from build123d import *

# Parameters (mm, degrees)
SCHIZZO4_R                   = 2.5
SCHIZZO4_R_2                 = 1.25
ESTRUSIONE_ESTRUSIONE3_DEPTH = 100
ESTRUSIONE_ESTRUSIONE4_DEPTH = 61.05
SCHIZZO6_W                   = 8.237008172
SCHIZZO6_H                   = 5.970383375
TAGLIO_ESTRUSIONE2_DEPTH     = 119.1
SCHIZZO7_W                   = 6.014694103
SCHIZZO7_H                   = 5.674261039
TAGLIO_ESTRUSIONE3_DEPTH     = 119.1
ESTRUSIONE_ESTRUSIONE5_REACH = 140.017
SCHIZZO8_W                   = 2.75
SCHIZZO8_H                   = 66.15
TAGLIO_ESTRUSIONE4_DEPTH     = 300
RACCORDO1_R                  = 2


with BuildPart() as part:
    # Schizzo4 → Estrusione-Estrusione3 (new body)
    with BuildSketch(Plane.XY):
        Circle(SCHIZZO4_R)
        Circle(SCHIZZO4_R_2, mode=Mode.SUBTRACT)
    extrude(amount=ESTRUSIONE_ESTRUSIONE3_DEPTH)

    # Schizzo5 → Estrusione-Estrusione4 (add, symmetric)
    with BuildSketch(Plane.XY.offset(50)):
        with BuildLine():
            Line((0, 2.5), (5, 2.5))
            Line((5, 2.5), (5, -64.15))
            Line((5, -64.15), (2.5, -64.15))
            Line((2.5, -64.15), (2.5, -2.5))
            Line((2.5, -2.5), (0, -2.5))
            ThreePointArc((0, -2.5), (2.5, 0), (0, 2.5))
        make_face()
    extrude(amount=ESTRUSIONE_ESTRUSIONE4_DEPTH, both=True)

    # Schizzo6 → Taglio-Estrusione2 (cut)
    with BuildSketch(Plane(origin=(0, 0, 0), x_dir=(-1, 0, 0), z_dir=(0, 0, -1))):
        with Locations((1.618504086, 0.485191688)):
            Rectangle(SCHIZZO6_W, SCHIZZO6_H)
    extrude(amount=TAGLIO_ESTRUSIONE2_DEPTH, mode=Mode.SUBTRACT)

    # Schizzo7 → Taglio-Estrusione3 (cut)
    with BuildSketch(Plane.XY.offset(100)):
        with Locations((-0.507347052, 0.33713052)):
            Rectangle(SCHIZZO7_W, SCHIZZO7_H)
    extrude(amount=TAGLIO_ESTRUSIONE3_DEPTH, mode=Mode.SUBTRACT)

    # Estrusione-Estrusione5: up to this face of the body (flat: up to its plane)
    estrusione_estrusione5_end = Plane(part.part.faces().sort_by_distance((3.75, -30.825, -11.05))[0])
    # Schizzo8 → Estrusione-Estrusione5 (add, up to the picked face)
    with BuildSketch(Plane.XY.offset(111.05), mode=Mode.PRIVATE) as estrusione_estrusione5_sk1:
        with Locations((3.625, -30.575)):
            Rectangle(SCHIZZO8_W, SCHIZZO8_H)
    estrusione_estrusione5_tool1 = split(extrude(estrusione_estrusione5_sk1.sketch, amount=-ESTRUSIONE_ESTRUSIONE5_REACH, mode=Mode.PRIVATE), bisect_by=estrusione_estrusione5_end, keep=Keep.BOTH, mode=Mode.PRIVATE)
    add(estrusione_estrusione5_tool1.solids().sort_by(Axis((3.625, -30.575, 111.05), (0, 0, -1)))[0])

    # Schizzo9 → Taglio-Estrusione4 (cut)
    with BuildSketch(Plane.XY.offset(100)):
        Polygon((2.25, -2.5), (2.25, -1.883948392), (1.619804847, -2.5), align=None)
    extrude(amount=-TAGLIO_ESTRUSIONE4_DEPTH, mode=Mode.SUBTRACT)

    # Raccordo1
    raccordo1_edges = [part.edges().sort_by_distance(p)[0] for p in [
        (1.619804847, -2.5, 50),
    ]]
    fillet(raccordo1_edges, radius=RACCORDO1_R)


solid = part.part
Work out the finished part from the listing and answer in its coordinate system (mm). A direction names the side the tool comes from. Coordinates: 2 decimals unless noted, no trailing zeros. Loops run counter-clockwise (first coordinate to the right, second up) from the corner with the lowest first, then second, coordinate; pieces in that order, holes last. Notation, with made-up numbers: M 82.25,-18 L 125.25,-18 A22 cw 125.25,5 Z; hole C -25,-39.75 d3. An arc over 180 degrees is marked long. Answer in a Markdown table with one row per item. Add a question column.
1. A tool of negligible diameter and unlimited length cuts with its end or side. For faces 1 (the cylindrical face through (-2.5, 0.1, 49.3)), 2 (the flat face through (-1, 1, 100)), 3 (the flat face through (-1, 1, 0)), from which of +Z, -Z, +X, -X, +Y, -Y can it reach the whole face along a straight path? Write none if from no direction.
2. Consider L1, parallel to Y at x = -0.25, z = 77; L2, parallel to X at y = -27, z = 1.5; L3, parallel to Y at x = -1, z = 64.5. Determine where each line is inside the solid, lowest interval first.
3. Find section C-C, the plane y = -43. Write down the section's boundary in (x, z).
4. The mould has two halves that part along X. Classify faces 4 (the flat face through (4, -30, -11.05)), 5 (the flat face through (5, -30, 51)), 6 (the cylindrical face through (-0.27, -1.22, 49.3)): pulls with the +X half, pulls with the -X half, needs draft (parallel to the pull), parting line crosses it, or undercut.
5. Find section B-B, the plane z = 87.5. Write down the section's boundary in (x, y), then the cut area to 3 significant figures.
6. Flat-ended cylindrical pins translate along their axes: P1, Ø0.6, axis at y = -64, z = 78, coming from the -X side; P2, Ø2, axis at x = 0, y = 0, coming from the -Z side; P3, Ø10, axis at y = -56, z = 8, coming from the -X side; P4, Ø1.4, axis at x = -1, y = 1, coming from the -Z side. Find the tip coordinate at first contact, or state that the pin passes through.
7. Find section A-A, the plane y = 0. Write down the section's boundary in (x, z).
Reported:
| question | item | result |
|---|---|---|
| 1 | face 1 | +Z, -Z, -X |
| 1 | face 2 | +Z, -X, +Y, -Y |
| 1 | face 3 | -Z, -X, +Y, -Y |
| 2 | L1 | y = -2.49 to -1.22, 1.22 to 2.49 |
| 2 | L2 | x = 2.25 to 5 |
| 2 | L3 | y = -2.29 to -0.75, 0.75 to 2.29 |
| 3 | outline | M 2.25,-11.05 L 5,-11.05 L 5,111.05 L 2.25,111.05 Z |
| 4 | face 4 | needs draft |
| 4 | face 5 | pulls with the +X half |
| 4 | face 6 | undercut |
| 5 | outline | M 0,-2.5 L 0.8,-2.5 A2 ccw 2.2,-1.93 L 2.25,-1.88 L 2.25,-63.65 L 2.5,-63.65 L 2.5,-64.15 L 5,-64.15 L 5,2.5 L 0,2.5 A2.5 ccw Z; hole C 0,0 d2.5 |
| 5 | area | 199 mm^2 |
| 6 | P1 | stops at x = 2.5 |
| 6 | P2 | passes through |
| 6 | P3 | stops at x = 2.25 |
| 6 | P4 | stops at z = 0 |
| 7 | outline | M -2.5,0 L -1.25,0 L -1.25,100 L -2.5,100 Z; M 1.25,0 L 2.25,0 L 2.25,-11.05 L 5,-11.05 L 5,111.05 L 2.25,111.05 L 2.25,100 L 1.25,100 Z |
